For this review, take the finished solid that the model builds, in its own axes (mm). Face numbers are marked on the shaded views. A direction names the side the tool comes from. Round coordinates to 2 decimals unless told otherwise and drop trailing zeros. Write each loop counter-clockwise with the first axis right and the second up, starting at its lowest first coordinate (ties: lowest second). Pieces come first, ordered by that corner, then holes. Notation, with made-up numbers: (-5.75, -28) -> (20.25, -28) arc R21 cw to (20.25, -15) -> close; hole circle Ø4 at (53, 9.25). An arc over 180 degrees is marked (long way). Answer as CSV lines item,"result". Start each with the question number.
Item 1: Take a section at D-D on z = 0.55. Give the boundary of the cut face in (x, y), then the cut area to 3 significant figures.
Item 2: Machinability: for the marked faces 1 and 2, which of the approach directions +Z, -Z, +X, -X, +Y, -Y give a long, thin tool a straight path to every point of the face, cutting with its end or side? Answer none if there is none.
Item 3: Wall thickness on probe 1 along Y at (x, z) = (0, 2.9); probe 2 along Y at (x, z) = (0, 1.7); probe 3 along X at (y, z) = (-6, 2.3): over which ranges is each line inside the solid? List them lowest first. Write a range as from..to.
Item 4: For pin 1 Ø3 at (x, y) = (0, 9.83) entering from -Z; pin 2 Ø2.5 at (y, z) = (-5, 1.5) entering from +X; pin 3 Ø12 at (x, y) = (8, -15.5) entering from +Z; pin 4 Ø2 at (x, z) = (16, 4) entering from +Y, all flat-tipped, find the tip position at first contact; note any pin that passes through.
Item 5: Take a section at A-A on x = -0.75. Give the boundary of the cut face in (y, z).
Item 6: Take a section at C-C on y = -20. Give the boundary of the cut face in (x, z).
Item 7: Take a section at B-B on y = -0.5. Give the boundary of the cut face in (x, z), then the cut area to 3 significant figures.
Item 8: Mouldability with a two-part tool opening along X and no side actions: class the marked faces 3, 4 and 5 as +X half, -X half, draft (parallel to the pull), parting line (faces both ways), or undercut.
```python
from build123d import *

# Parameters (mm, degrees)
F1_DEPTH = 2
F2_DEPTH = 5
F3_D     = 3.5


with BuildPart() as f1:
    # F0 (on Top) → F1 (new body)
    with BuildSketch(Plane.XY):
        with BuildLine():
            Line((10.0519920066, -31.4581375476), (17.1230598185, -24.3870697357))
            Line((17.1230598185, -24.3870697357), (15.7088462561, -22.9728561734))
            Line((15.7088462561, -22.9728561734), (7.4758086988, -14.739818616))
            Line((7.4758086988, -14.739818616), (1.6548871607, -8.918897078))
            Line((1.6548871607, -8.918897078), (0.9610006781, -8.2250105953))
            ThreePointArc((0.9610006781, -8.2250105953), (-0.4532128843, -7.6392241577), (-1.8674264467, -8.2250105953))
            Line((-1.8674264467, -8.2250105953), (-6.1100671338, -12.4676512825))
            ThreePointArc((-6.1100671338, -12.4676512825), (-6.6958535714, -13.8818648448), (-6.1100671338, -15.2960784072))
            Line((-6.1100671338, -15.2960784072), (-4.0901436171, -17.3160019239))
            Line((-4.0901436171, -17.3160019239), (8.6377784442, -30.0439239852))
            Line((8.6377784442, -30.0439239852), (10.0519920066, -31.4581375476))
        make_face()
    extrude(amount=F1_DEPTH)

    # F0 (on Top) → F2 (join)
    with BuildSketch(Plane.XY):
        with BuildLine():
            Line((8.8900222611, -13.3256050537), (9, -13.3256050537))
            Line((9, -13.3256050537), (9, 11.3256050537))
            ThreePointArc((9, 11.3256050537), (8.4142135624, 12.739818616), (7, 13.3256050537))
            Line((7, 13.3256050537), (-7, 13.3256050537))
            ThreePointArc((-7, 13.3256050537), (-8.4142135624, 12.739818616), (-9, 11.3256050537))
            Line((-9, 11.3256050537), (-9, -13.3256050537))
            Line((-9, -13.3256050537), (-9, -15.2345726658))
            Line((-9, -15.2345726658), (-5.5043571795, -18.7302154863))
            Line((-5.5043571795, -18.7302154863), (8.6377784442, -32.87235111))
            Line((8.6377784442, -32.87235111), (10.0519920066, -31.4581375476))
            Line((10.0519920066, -31.4581375476), (8.6377784442, -30.0439239852))
            Line((8.6377784442, -30.0439239852), (-4.0901436171, -17.3160019239))
            Line((-4.0901436171, -17.3160019239), (-6.1100671338, -15.2960784072))
            ThreePointArc((-6.1100671338, -15.2960784072), (-6.6958535714, -13.8818648448), (-6.1100671338, -12.4676512825))
            Line((-6.1100671338, -12.4676512825), (-1.8674264467, -8.2250105953))
            ThreePointArc((-1.8674264467, -8.2250105953), (-0.4532128843, -7.6392241577), (0.9610006781, -8.2250105953))
            Line((0.9610006781, -8.2250105953), (1.6548871607, -8.918897078))
            Line((1.6548871607, -8.918897078), (7.4758086988, -14.739818616))
            Line((7.4758086988, -14.739818616), (15.7088462561, -22.9728561734))
            Line((15.7088462561, -22.9728561734), (17.1230598185, -24.3870697357))
            Line((17.1230598185, -24.3870697357), (18.5372733808, -22.9728561734))
            Line((18.5372733808, -22.9728561734), (8.8900222611, -13.3256050537))
        make_face()
    extrude(amount=F2_DEPTH)

    # F3 (through all)
    with Locations(Plane(origin=(0, 0, 0), x_dir=(1, 0, 0), z_dir=(0, 0, -1))):
        with Locations((0, -0.5559050478), (-0.9101199103, 13.4369833395), (0, -9.8313745111)):
            Hole(F3_D / 2)


solid = f1.part
```
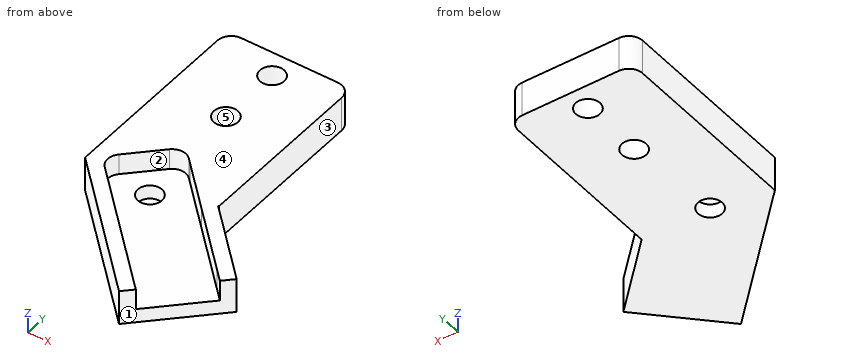
Output values:
1,outline,"(-9, -15.23) -> (8.64, -32.87) -> (18.54, -22.97) -> (8.89, -13.33) -> (9, -13.33) -> (9, 11.33) arc R2 ccw to (7, 13.33) -> (-7, 13.33) arc R2 ccw to (-9, 11.33) -> close; hole circle Ø3.5 at (-0.91, -13.44); hole circle Ø3.5 at (0, 0.56); hole circle Ø3.5 at (0, 9.83)"
1,area,"736 mm^2"
2,face 1,"+Z, -Z, +X, -Y"
2,face 2,"+Z"
3,probe 1,"y = -24.23..-21.41, -7.69..-1.19, 2.31..8.08, 11.58..13.33"
3,probe 2,"y = -24.23..-14.93, -11.94..-1.19, 2.31..8.08, 11.58..13.33"
3,probe 3,"x = -9..9"
4,pin 1,"passes through"
4,pin 2,"stops at x = 9"
4,pin 3,"stops at z = 5"
4,pin 4,"stops at y = -19.44"
5,outline,"(-23.48, 0) -> (-15.18, 0) -> (-15.18, 2) -> (-20.66, 2) -> (-20.66, 5) -> (-23.48, 5) -> close; (-11.69, 0) -> (-1.03, 0) -> (-1.03, 5) -> (-7.66, 5) -> (-7.66, 2) -> (-11.69, 2) -> close; (2.14, 0) -> (8.25, 0) -> (8.25, 5) -> (2.14, 5) -> close; (11.41, 0) -> (13.33, 0) -> (13.33, 5) -> (11.41, 5) -> close"
6,outline,"(-4.23, 0) -> (15.56, 0) -> (15.56, 5) -> (12.74, 5) -> (12.74, 2) -> (-1.41, 2) -> (-1.41, 5) -> (-4.23, 5) -> close"
7,outline,"(-9, 0) -> (-1.4, 0) -> (-1.4, 5) -> (-9, 5) -> close; (1.4, 0) -> (9, 0) -> (9, 5) -> (1.4, 5) -> close"
7,area,"76.0 mm^2"
8,face 3,"+X half"
8,face 4,"draft"
8,face 5,"undercut"
